Here's how the part is built. I have some questions about the finished solid (model axes, mm). Face numbers are marked on the shaded views. A direction names the side the tool comes from. Round coordinates to 2 decimals unless told otherwise and drop trailing zeros. Order: outer loops, then holes, each group sorted by start corner. A loop starts at its lowest first (then second) coordinate and runs counter-clockwise, first axis right, second up. Notation, with made-up numbers: M -24.75,8 L 9.25,8 A11 cw 9.25,21 Z; hole C -29.75,17 d8. An arc over 180 degrees is marked long. Use one line per item in the form item = value. Start each with the question number.
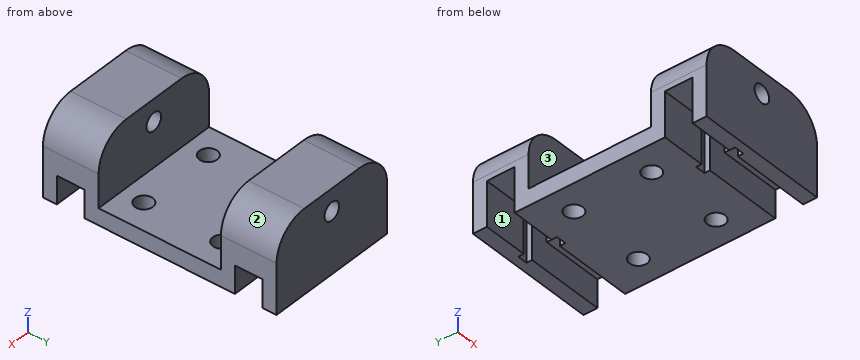
```python
from build123d import *

# Parameters (mm, degrees)
CYLINDER171_R     = 1.6
CYLINDER171_DEPTH = 10
CYLINDER173_R     = 1.6
CYLINDER173_DEPTH = 10
CYLINDER172_R     = 1.6
CYLINDER172_DEPTH = 10
CYLINDER170_R     = 1.6
CYLINDER170_DEPTH = 10
CYLINDER169_R     = 1.6
CYLINDER169_DEPTH = 10
BOX090_W          = 19
BOX090_H          = 5
BOX090_DEPTH      = 5
BOX089_W          = 4
BOX089_H          = 5
BOX089_DEPTH      = 8
BOX088_W          = 1.8
BOX088_H          = 7
BOX088_DEPTH      = 11
BOX086_W          = 8
BOX086_H          = 5
BOX086_DEPTH      = 8
BOX087_W          = 24
BOX087_H          = 10
BOX087_DEPTH      = 15
FILLET048_R       = 6
BOX091_W          = 24
BOX091_H          = 22
BOX091_DEPTH      = 3
FILLET047_R       = 6


with BuildPart() as cylinder171:
    # Cylinder171 → Cylinder171 (new body)
    with BuildSketch(Plane(origin=(50, 24, 12), x_dir=(1, 0, 0), z_dir=(0, 0, 1))):
        Circle(CYLINDER171_R)
    extrude(amount=CYLINDER171_DEPTH)


with BuildPart() as cylinder173:
    # Cylinder173 → Cylinder173 (new body)
    with BuildSketch(Plane(origin=(64, 24, 12), x_dir=(1, 0, 0), z_dir=(0, 0, 1))):
        Circle(CYLINDER173_R)
    extrude(amount=CYLINDER173_DEPTH)


with BuildPart() as cylinder172:
    # Cylinder172 → Cylinder172 (new body)
    with BuildSketch(Plane(origin=(64, 38, 12), x_dir=(1, 0, 0), z_dir=(0, 0, 1))):
        Circle(CYLINDER172_R)
    extrude(amount=CYLINDER172_DEPTH)


with BuildPart() as fusion152:
    # Cylinder170 → Cylinder170 (new body)
    with BuildSketch(Plane(origin=(50, 38, 12), x_dir=(1, 0, 0), z_dir=(0, 0, 1))):
        Circle(CYLINDER170_R)
    extrude(amount=CYLINDER170_DEPTH)

    # Fusion152: union Cylinder171, Cylinder173, Cylinder172
    add(cylinder171.part)
    add(cylinder173.part)
    add(cylinder172.part)


with BuildPart() as cylinder169:
    # Cylinder169 → Cylinder169 (new body)
    with BuildSketch(Plane(origin=(57, 52, 30), x_dir=(1, 0, 0), z_dir=(0, -1, 0))):
        Circle(CYLINDER169_R)
    extrude(amount=CYLINDER169_DEPTH)


with BuildPart() as cube058:
    # Box090 → Box090 (new body)
    with BuildSketch(Plane(origin=(54, 44.5, 19), x_dir=(1, 0, 0), z_dir=(0, 0, 1))):
        with Locations((9.5, 2.5)):
            Rectangle(BOX090_W, BOX090_H)
    extrude(amount=BOX090_DEPTH)


with BuildPart() as cube057:
    # Box089 → Box089 (new body)
    with BuildSketch(Plane(origin=(54, 44.5, 19), x_dir=(1, 0, 0), z_dir=(0, 0, 1))):
        with Locations((2, 2.5)):
            Rectangle(BOX089_W, BOX089_H)
    extrude(amount=BOX089_DEPTH)


with BuildPart() as cube056:
    # Box088 → Box088 (new body)
    with BuildSketch(Plane(origin=(53, 43.5, 19), x_dir=(1, 0, 0), z_dir=(0, 0, 1))):
        with Locations((0.9, 3.5)):
            Rectangle(BOX088_W, BOX088_H)
    extrude(amount=BOX088_DEPTH)


with BuildPart() as cube054:
    # Box086 → Box086 (new body)
    with BuildSketch(Plane(origin=(45, 44.5, 19), x_dir=(1, 0, 0), z_dir=(0, 0, 1))):
        with Locations((4, 2.5)):
            Rectangle(BOX086_W, BOX086_H)
    extrude(amount=BOX086_DEPTH)


with BuildPart() as cut106:
    # Box087 → Box087 (new body)
    with BuildSketch(Plane(origin=(45, 42, 19), x_dir=(1, 0, 0), z_dir=(0, 0, 1))):
        with Locations((12, 5)):
            Rectangle(BOX087_W, BOX087_H)
    extrude(amount=BOX087_DEPTH)

    # Cut103: cut Cube054
    add(cube054.part, mode=Mode.SUBTRACT)

    # Cut104: cut Cube056
    add(cube056.part, mode=Mode.SUBTRACT)

    # Cut105: cut Cube057
    add(cube057.part, mode=Mode.SUBTRACT)

    # Cut106: cut Cube058
    add(cube058.part, mode=Mode.SUBTRACT)


with BuildPart() as fillet048:
    # Cut108 base: copy of Cut106
    add(cut106.part)

    # Cut108: cut Cylinder169
    add(cylinder169.part, mode=Mode.SUBTRACT)

    # Fillet048
    fillet048_edges = [fillet048.edges().sort_by_distance(p)[0] for p in [
        (45, 47, 34),
        (69, 47, 34),
    ]]
    fillet(fillet048_edges, radius=FILLET048_R)


with BuildPart() as cube059:
    # Box091 → Box091 (new body)
    with BuildSketch(Plane(origin=(45, 20, 19), x_dir=(1, 0, 0), z_dir=(0, 0, 1))):
        with Locations((12, 11)):
            Rectangle(BOX091_W, BOX091_H)
    extrude(amount=BOX091_DEPTH)


with BuildPart() as fake_cylinder_holder:
    # Cut107 base: copy of Cut106
    add(cut106.part)

    # Cut107: cut Cylinder169
    add(cylinder169.part, mode=Mode.SUBTRACT)

    # Fillet047
    fillet047_edges = [fake_cylinder_holder.edges().sort_by_distance(p)[0] for p in [
        (45, 47, 34),
        (69, 47, 34),
    ]]
    fillet(fillet047_edges, radius=FILLET047_R)


with BuildPart() as fake_cylinder_holder_1:
    # Fillet047 placement: moved
    add(fake_cylinder_holder.part.moved(Location((0, -32, 0))))

    # Fusion151: union Fillet048, Cube059
    add(fillet048.part)
    add(cube059.part)

    # Cut110: cut Fusion152
    add(fusion152.part, mode=Mode.SUBTRACT)


solid = fake_cylinder_holder_1.part
```
1) If we section it at B-B on y = 38: Write out the boundary of the cut face in (x, z).
2) If we section it at A-A on x = 57: Write out the boundary of the cut face in (y, z), then the cut area to 3 significant figures.
3) Will these pins go through, and if not, where does the flat tip stop? pin 1 Ø0.9 at (y, z) = (15.5, 26) entering from -X; pin 2 Ø1.5 at (x, y) = (49, 18.5) entering from +Z; pin 3 Ø1.6 at (x, y) = (57, 46) entering from -Z; pin 4 Ø3 at (x, z) = (57, 30) entering from -Y.
4) On a 3-axis mill with a long thin cutter (end or side, diameter ignored), from which of +Z, -Z, +X, -X, +Y, -Y can I reach the whole of each face in a straight line? I mean the marked faces 1, 2 and 3. Say none if no direction works.
5) If we section it at C-C on z = 20.75: Give the number of separate pieces and of enclosed holes in the cut face, then the cut area to 3 significant figures.
6) If I drill on line 1 (Y direction, x = 53.5, z = 23.5); line 2 (X direction, y = 24, z = 20.9); line 3 (Y direction, x = 51, z = 26.75), over which ranges is the centre line in solid material (lowest first)?
Completed:
q1.outline = M 45,19 L 48.4,19 L 48.4,22 L 45,22 Z; M 51.6,19 L 62.4,19 L 62.4,22 L 51.6,22 Z; M 65.6,19 L 69,19 L 69,22 L 65.6,22 Z
q2.outline = M 10,19 L 12.5,19 L 12.5,27 L 17.5,27 L 17.5,19 L 44.5,19 L 44.5,27 L 49.5,27 L 49.5,19 L 52,19 L 52,28.4 L 42,28.4 L 42,22 L 20,22 L 20,28.4 L 10,28.4 Z; M 10,31.6 L 20,31.6 L 20,34 L 10,34 Z; M 42,31.6 L 52,31.6 L 52,34 L 42,34 Z
q2.area = 222 mm²
q3.pin_1 = 58
q3.pin_2 = 33.87
q3.pin_3 = 27
q3.pin_4 = through
q4.face_1 = -Z, -X
q4.face_2 = +Z, +X, +Y, -Y
q4.face_3 = +Z, +X, -X
q5.separate_pieces = 3
q5.enclosed_holes = 4
q5.area = 729 mm²
q6.line_1 = 10 to 11.5, 18.5 to 20, 42 to 43.5, 50.5 to 52
q6.line_2 = 45 to 48.4, 51.6 to 62.4, 65.6 to 69
q6.line_3 = 10 to 12.5, 17.5 to 20, 42 to 44.5, 49.5 to 52
